from build123d import *

# Parameters (mm, degrees)
SKETCH_1_W          = 130
SKETCH_1_H          = 130
EXTRUDE_1_DEPTH     = 139
SKETCH_2_R          = 55
EXTRUDE_2_DEPTH     = 6
SKETCH_3_R          = 11
EXTRUDE_3_DEPTH     = 52
SKETCH_5_R          = 4.5
CUT_EXTRUDE_2_DEPTH = 137
CUT_EXTRUDE_5_DEPTH = 221.093162093
SKETCH_10_OUTSIDE_W = 185.892
SKETCH_10_OUTSIDE_H = 185.892
SKETCH_10_OUTSIDE_R = 82.5
CUT_EXTRUDE_6_DEPTH = 231.479934051


with BuildPart() as part:
    # 草图1 → 拉伸1 (new body)
    with BuildSketch(Plane.XY):
        with Locations((65, -65)):
            Rectangle(SKETCH_1_W, SKETCH_1_H)
    extrude(amount=EXTRUDE_1_DEPTH)

    # 草图2 → 拉伸2 (add)
    with BuildSketch(Plane(origin=(0, 0, 0), x_dir=(-1, 0, 0), z_dir=(0, 0, -1))):
        with Locations(Location((-65, -65, 0), (0, 0, 180))):
            Circle(SKETCH_2_R)
    extrude(amount=EXTRUDE_2_DEPTH)

    # 草图3 → 拉伸3 (add)
    with BuildSketch(Plane(origin=(0, 0, -6), x_dir=(-1, 0, 0), z_dir=(0, 0, -1))):
        with Locations(Location((-65, -65, 0), (0, 0, 180))):
            Circle(SKETCH_3_R)
    extrude(amount=EXTRUDE_3_DEPTH)

    # 草图5 → 切除-拉伸2 (cut)
    with BuildSketch(Plane(origin=(0, 0, 0), x_dir=(-1, 0, 0), z_dir=(0, 0, -1))):
        with Locations((-13.734758364, -13.734758364)):
            Circle(SKETCH_5_R)
        with Locations((-13.734758364, -116.265241636)):
            Circle(SKETCH_5_R)
        with Locations((-116.265241636, -116.265241636)):
            Circle(SKETCH_5_R)
        with Locations((-116.265241636, -13.734758364)):
            Circle(SKETCH_5_R)
    extrude(amount=-CUT_EXTRUDE_2_DEPTH, mode=Mode.SUBTRACT)

    # 草图7 → 切除-拉伸5 (cut, through all)
    with BuildSketch(Plane(origin=(0, 0, 18), x_dir=(-1, 0, 0), z_dir=(0, 0, -1))):
        with BuildLine():
            Line((-130, 0), (-105, 0))
            Line((-105, 0), (-105, -10))
            ThreePointArc((-105, -10), (-109.393398282, -20.606601718), (-120, -25))
            Line((-120, -25), (-130, -25))
            Line((-130, -25), (-130, 0))
        make_face()
        with BuildLine():
            Line((0, 0), (0, -25))
            Line((0, -25), (-10, -25))
            ThreePointArc((-10, -25), (-20.606601718, -20.606601718), (-25, -10))
            Line((-25, -10), (-25, 0))
            Line((-25, 0), (0, 0))
        make_face()
        with BuildLine():
            Line((0, -130), (-25, -130))
            Line((-25, -130), (-25, -120))
            ThreePointArc((-25, -120), (-20.606601718, -109.393398282), (-10, -105))
            Line((-10, -105), (0, -105))
            Line((0, -105), (0, -130))
        make_face()
        with BuildLine():
            Line((-130, -130), (-130, -105))
            Line((-130, -105), (-120, -105))
            ThreePointArc((-120, -105), (-109.393398282, -109.393398282), (-105, -120))
            Line((-105, -120), (-105, -130))
            Line((-105, -130), (-130, -130))
        make_face()
    extrude(amount=-CUT_EXTRUDE_5_DEPTH, mode=Mode.SUBTRACT)

    # 草图10 outside → 切除-拉伸6 (cut, through all)
    with BuildSketch(Plane(origin=(0, 0, 0), x_dir=(-1, 0, 0), z_dir=(0, 0, -1))):
        with Locations((-65, -65)):
            Rectangle(SKETCH_10_OUTSIDE_W, SKETCH_10_OUTSIDE_H)
        with Locations((-65, -65)):
            Circle(SKETCH_10_OUTSIDE_R, mode=Mode.SUBTRACT)
    extrude(amount=-CUT_EXTRUDE_6_DEPTH, mode=Mode.SUBTRACT)


solid = part.part
Model file for the job. Use its own axes, mm. A direction names the side the tool comes from. Round coordinates to 2 decimals unless told otherwise and drop trailing zeros. Loops run counter-clockwise (first coordinate to the right, second up) from the corner with the lowest first, then second, coordinate; pieces in that order, holes last. Notation, with made-up numbers: M 78,30.5 L 115,30.5 A28 cw 115,52.5 Z; hole C 87.25,2 d1. An arc over 180 degrees is marked long. One line per question, with ' | ' between items.
1) Band-saw the part on D-D (x = 80.5). Give the cut face in (y, z), then the cut area to 3 significant figures.
Solved:
outline: M -130,0 L -117.77,0 L -117.77,-6 L -12.23,-6 L -12.23,0 L 0,0 L 0,139 L -130,139 Z | area: 18,700 mm²
2) 3-axis set-ups, long thin cutter, end or side, ignore diameter. For faces 5 (the cylindrical face through (20.49, -20.72, 77.65)), 6 (the cylindrical face through (56.89, -72.43, -31.64)), 7 (the cylindrical face through (20.72, -109.51, 77.65)), 8 (the flat face through (120, -120, 18)), 9 (the flat face through (120, -10, 18)): which of +Z, -Z, +X, -X, +Y, -Y reach the whole face in a straight line?
Solved:
face 5: +Z, -X, +Y | face 6: -Z | face 7: +Z, -X, -Y | face 8: +Z, +X, -Y | face 9: +Z, +X, +Y
3) Band-saw the part on C-C (y = -65). Give the cut face in (x, z).
Solved:
outline: M 0,0 L 10,0 L 10,-6 L 54,-6 L 54,-58 L 76,-58 L 76,-6 L 120,-6 L 120,0 L 130,0 L 130,139 L 0,139 Z
4) Band-saw the part on B-B (x = 65). Give the cut face in (y, z), then the cut area to 3 significant figures.
Solved:
outline: M -130,0 L -120,0 L -120,-6 L -76,-6 L -76,-58 L -54,-58 L -54,-6 L -10,-6 L -10,0 L 0,0 L 0,139 L -130,139 Z | area: 19,900 mm²
5) Band-saw the part on A-A (z = 80.5). Give the cut face in (x, y).
Solved:
outline: M 0,-105 L 10,-105 A15 cw 25,-120 L 25,-130 L 105,-130 L 105,-120 A15 cw 120,-105 L 130,-105 L 130,-25 L 120,-25 A15 cw 105,-10 L 105,0 L 25,0 L 25,-10 A15 cw 10,-25 L 0,-25 Z
6) Drill centre lines: line 1 along Z through (x, y) = (113.5, -40.5); line 2 along X through (y, z) = (-119.5, 45); line 3 along Z through (x, y) = (29, -9). Where is each one in solid material? Low to high.
Solved:
line 1: z = -6 to 139 | line 2: x = 24.99 to 105.01 | line 3: z = 0 to 139
7) Mould opens along X. For faces 1 (the flat face through (64, 0, 69)), 2 (the cylindrical face through (112.11, -117.99, 8.87)), 3 (the cylindrical face through (11.66, -120.26, 8.87)), 4 (the cylindrical face through (109.51, -109.28, 77.65)) say: +X half, -X half, draft (parallel to the pull), parting line (faces both ways), or undercut.
Solved:
face 1: draft | face 2: undercut | face 3: undercut | face 4: +X half
8) Flat gauge pins, fed straight in: pin 1 (8 mm diameter, centred on y = -3.5, z = 76, fed in from +X); pin 2 (3 mm diameter, centred on y = -127.5, z = 106.5, fed in from -X); pin 3 (11 mm diameter, centred on x = 5.5, z = 56, fed in from -Y). Where does each tip first touch, or does it go through?
Solved:
pin 1: stops at x = 105 | pin 2: stops at x = 25 | pin 3: stops at y = -105.03
